Job drawing, mm, ordinate dimensions from the low corner. One solid piece. Give positions to 0.01 mm unless a question says otherwise; leave off trailing zeros. Write each loop counter-clockwise with the first axis right and the second up, starting at its lowest first coordinate (ties: lowest second). Pieces come first, ordered by that corner, then holes. Notation, with made-up numbers: (-11.5, -16.75) - (40.5, -16.75) arc R34 cw to (40.5, 17.25) - close; hole circle Ø10 at (-37.5, 20.5). An arc over 180 degrees is marked (long way). Answer in a Markdown table with one row per item. Add a question column.
1. Band-saw the part on B-B on y = 5. Write the cut outline in (x, z).
2. Band-saw the part on C-C on z = 4.5. Write the cut outline in (x, y), plus the area to 3 significant figures.
3. Drop a flat-ended pin along its axis: pin 1 Ø6 at (x, z) = (15.5, 7.5) entering from -Y. Give the stop position or say it passes through.
4. Band-saw the part on A-A on x = 5. Write the cut outline in (y, z).
5. Pull direction X, two halves, no side cores. Call the marked faces 1, 2, 3 and 4: released by +X, released by -X, zero draft, split by the parting line, or undercut.
6. Probe line 1 along Y through (x, z) = (5, 3.5); line 2 along X through (y, z) = (14.5, 3.25); line 3 along Y through (x, z) = (18, 5.5). List the from-to ranges inside material, lowest first.
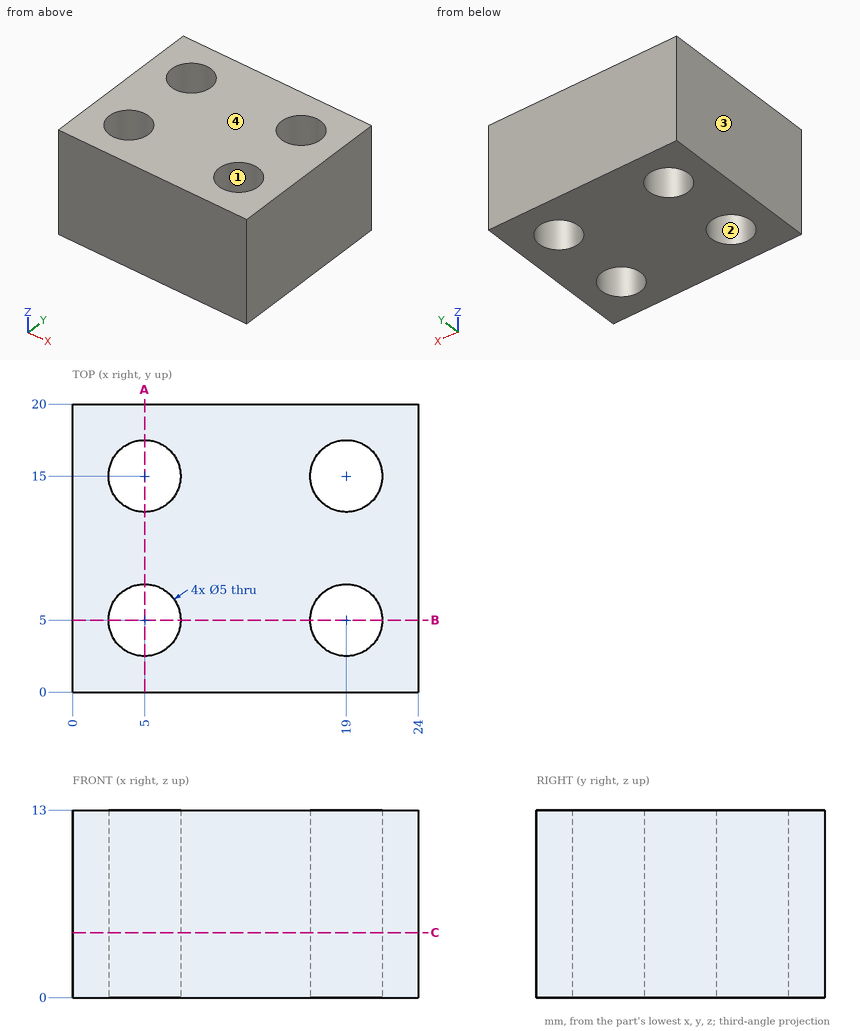
Values:
| question | item | result |
|---|---|---|
| 1 | outline | (0, 0) - (2.5, 0) - (2.5, 13) - (0, 13) - close; (7.5, 0) - (16.5, 0) - (16.5, 13) - (7.5, 13) - close; (21.5, 0) - (24, 0) - (24, 13) - (21.5, 13) - close |
| 2 | outline | (0, 0) - (24, 0) - (24, 20) - (0, 20) - close; hole circle Ø5 at (5, 5); hole circle Ø5 at (5, 15); hole circle Ø5 at (19, 5); hole circle Ø5 at (19, 15) |
| 2 | area | 401 mm² |
| 3 | pin 1 | stops at y = 0 |
| 4 | outline | (0, 0) - (2.5, 0) - (2.5, 13) - (0, 13) - close; (7.5, 0) - (12.5, 0) - (12.5, 13) - (7.5, 13) - close; (17.5, 0) - (20, 0) - (20, 13) - (17.5, 13) - close |
| 5 | face 1 | undercut |
| 5 | face 2 | undercut |
| 5 | face 3 | released by -X |
| 5 | face 4 | zero draft |
| 6 | line 1 | y = 0 to 2.5, 7.5 to 12.5, 17.5 to 20 |
| 6 | line 2 | x = 0 to 2.55, 7.45 to 16.55, 21.45 to 24 |
| 6 | line 3 | y = 0 to 2.71, 7.29 to 12.71, 17.29 to 20 |
